Autodesk Inventor part; units mm, degrees
ref_plane "Work Plane3" through (0, 22.5, 0) normal (0, 1, 0) x (1, 0, 0)
ref_plane "YZ Plane" through (0, 0, 0) normal (1, 0, 0) x (0, 1, 0)
ref_plane "XZ Plane" through (0, 0, 0) normal (0, 1, 0) x (-1, 0, 0)
sketch "Sketch1" plane through (0, 0, 0) normal (0, 1, 0) x (-1, 0, 0)
  line L0 (-67.5, 75) -> (67.5, 75)
  line L1 (67.5, 75) -> (67.5, -75)
  line L2 (67.5, -75) -> (-67.5, -75)
  line L3 (-67.5, -75) -> (-67.5, 75)
  line L4 (-67.5, 75) -> (67.5, -75) construction
  line L5 (67.5, 75) -> (-67.5, -75) construction
  point P0 (0, 0)
  dimension "d0" = 135
  dimension "d1" = 150
extrude "Extrusion1" add sketch "Sketch1" along normal blind 8
sketch "Sketch3" plane through (0, 8, 0) normal (0, 1, 0) x (1, 0, 0)
  line L0 (-67.5, -75) -> (67.5, -75)
  line L1 (67.5, -75) -> (67.5, 75)
  line L2 (67.5, 75) -> (-67.5, 75)
  line L3 (-67.5, 75) -> (-67.5, -75)
  line L4 (62.5, 75) -> (62.5, -70)
  line L5 (-67.5, -75) -> (67.5, -75)
  line L6 (67.5, -75) -> (67.5, 75)
  line L7 (0, 0) -> (0, -83) construction
  line L8 (-62.5, 75) -> (-62.5, -70)
  line L9 (62.5, -70) -> (-62.5, -70)
  dimension "d4" = 5
  dimension "d5" = 5
extrude "Extrusion2" add sketch "Sketch3" along normal blind 20 contours L3 L2 L8 L9 L4 L1 L0
sketch "Sketch4" plane through (67.5, 0, -75) normal (0, 0, -1) x (-1, 0, 0)
  line L0 (135, 0) -> (0, 0)
  line L1 (135, 0) -> (135, 28)
  line L2 (130, 28) -> (135, 28)
  line L3 (130, 8) -> (130, 28)
  line L4 (5, 8) -> (130, 8)
  line L5 (5, 8) -> (5, 28)
  line L6 (0, 28) -> (5, 28)
  line L7 (0, 0) -> (0, 28)
  line L8 (130, 8) -> (5, 8)
  line L9 (5, 8) -> (5, 0)
  line L10 (130, 8) -> (130, 0)
  line L11 (0, 0) -> (135, 0)
  line L12 (0, 0) -> (0, 28)
  line L13 (5, 0) -> (130, 0)
  line L14 (5, 8) -> (130, 8)
  line L15 (5, 4) -> (130, 4)
  line L16 (5, 8) -> (0, 8)
  line L17 (135, 0) -> (0, 0)
  point P0 (67.5, 0)
  dimension "d8" = 0
  dimension "d9" = 4
extrude "Extrusion3" add sketch "Sketch4" along normal blind 20 contours L0 L10 L3 L2 L1 | L0 L9 L15 L10 | L15 L9 L4 L10 | L7 L6 L5 L16
sketch "Sketch6" plane through (67.5, 0, 75) normal (1, 0, 0) x (0, 0, -1)
  line L0 (150, 0) -> (150, 8)
  line L1 (0, 0) -> (0, 28)
  line L2 (170, 18) -> (157, 18)
  line L3 (157, 18) -> (157, 28)
  line L4 (157, 28) -> (170, 28)
  line L5 (170, 28) -> (170, 18)
  line L6 (170, 28) -> (170, 8)
  line L7 (150, 8) -> (170, 8)
  line L8 (0, 28) -> (170, 28)
  point P0 (75, 0)
  dimension "d83" = 10
  dimension "d85" = 10
  dimension "d86" = 0
  dimension "d87" = 13
  dimension "d88" = 0
  dimension "d89" = 0
extrude "Extrusion4" cut sketch "Sketch6" against normal through all
fillet "Fillet1" radius 2 11 edges at (67.5, 0, 0) (67.5, 28, -3.5) (67.5, 14, 75) (0, 28, 75) (0, 0, 75) (-67.5, 28, -3.5) (-67.5, 14, 75) (-67.5, 0, -10) (62.5, 28, -6) (-62.5, 28, -6) (0, 28, 70)
sketch "Sketch11" plane through (-67.5, 9.7, -88) normal (-1, 0, 0) x (0, 0, 1)
  line L0 (9, 17.5) -> (0, 19.5)
  line L1 (0, 19.5) -> (0, 11.5)
  line L2 (0, 11.5) -> (9, 14)
  line L3 (9, 17.5) -> (9, 14)
  line L4 (9, 6) -> (0, 8.5)
  line L5 (0, 0) -> (9, 2.5)
  line L6 (0, 6) -> (0, 0)
  line L7 (9, 6) -> (9, 2.5)
  point P0 (88, -9.7)
sketch "Sketch12" plane through (-67.5, 2, 73) normal (-1, 0, 0) x (0, 0, 1)
  line L0 (-168, 28) -> (-168, 20)
  line L1 (-159, 26) -> (-168, 28)
  line L2 (-159, 26) -> (-159, 22.5)
  line L3 (-168, 20) -> (-159, 22.5)
  line L4 (-168, 17) -> (-168, 8.5)
  line L5 (-159, 14.5) -> (-168, 17)
  line L6 (-159, 14.5) -> (-159, 11)
  line L7 (-168, 8.5) -> (-159, 11)
  line L8 (-168, 0) -> (-168, 16)
  line L9 (-161, 19.2) -> (-161, 27.2)
  line L10 (-161, 27.2) -> (-168, 27.2)
  line L11 (-168, 16) -> (-168, 6)
  line L12 (-159, 17) -> (-168, 17)
  point P0 (-73, -2)
  point P1 (-168, 24)
sketch "Sketch15" plane through (62.5, 6, -75) normal (1, 0, 0) x (0, 0, -1)
  line L0 (0, -6) -> (0, 2)
  line L1 (20, 2) -> (20, -6)
  line L2 (0, 2) -> (20, 2)
  line L3 (0, -6) -> (20, -6)
  point P0 (-75, -6)
extrude "Extrusion8" add sketch "Sketch15" along normal blind 2.5
sketch "Sketch16" plane through (0, 8, 0) normal (0, 1, 0) x (1, 0, 0)
  line L0 (-62.5, -35) -> (-52.5, -35)
  line L1 (-52.5, -35) -> (-52.5, 5)
  line L2 (-52.5, 5) -> (-62.5, 5)
  line L3 (-62.5, 5) -> (-62.5, -35)
  line L4 (62.5, -70) -> (-62.5, -70)
  line L5 (-62.5, -70) -> (-62.5, 82)
  line L6 (51.5, -70) -> (62.5, -70)
  line L7 (62.5, -70) -> (62.5, -30)
  line L8 (62.5, -30) -> (51.5, -30)
  line L9 (51.5, -30) -> (51.5, -70)
  line L10 (62.5, 82) -> (62.5, -70)
  point P0 (0, 0)
  point P1 (-62.5, 95)
  point P2 (62.5, 95)
  dimension "d39" = 35
  dimension "d40" = 0
  dimension "d41" = 10
  dimension "d42" = 40
  dimension "d43" = 0
  dimension "d44" = 0
  dimension "d45" = 40
  dimension "d46" = 11
extrude "Extrusion9" add sketch "Sketch16" along normal blind 16
fillet "Fillet4" radius 1 8 edges at (51.5, 24, 50) (57, 24, 30) (51.5, 16, 30) (-52.5, 24, 15) (-52.5, 16, -5) (-57.5, 24, 35) (-57.5, 24, -5) (-52.5, 16, 35)
sketch "Sketch17" plane through (0, 24, 0) normal (0, 1, 0) x (1, 0, 0)
  circle A0 centre (-59, -25) radius 2.25
  line L0 (-62.5, -34) -> (-62.5, 4)
  line L1 (-53.5, -34) -> (-62.5, -34)
  circle A1 centre (58.5, -57.5) radius 2.25
  line L2 (52.5, -70) -> (52.5, -31)
  line L3 (52.5, -31) -> (62.5, -31)
  line L4 (62.5, -70) -> (50.5, -70)
  point P0 (0, 0)
  dimension "d50" = 4.5
  dimension "d51" = 3.5
  dimension "d52" = 9
  dimension "d53" = 4.5
  dimension "d54" = 6
  dimension "d90" = 12.5
extrude "Extrusion10" cut sketch "Sketch17" against normal blind 12
sketch "Sketch18" plane through (-62.5, 9.7, -88) normal (1, 0, 0) x (0, 0, -1)
  circle A0 centre (-68, 13.3) radius 2.25
  circle A1 centre (-37.2, 13.3) radius 2.25
  line L0 (0, 8.1) -> (0, 14.1)
  line L1 (-37.2, 13.3) -> (-68, 13.3)
  line L2 (-6, 18.3) -> (-160, 18.3)
  line L3 (-158, -1.7) -> (-158, 16.3)
  point P0 (-88, -9.7)
  point P1 (7, 18.3)
  dimension "d60" = 4.5
  dimension "d61" = 4.5
  dimension "d62" = 30.8
  dimension "d64" = 5
  dimension "d67" = 90
extrude "Extrusion11" cut sketch "Sketch18" against normal through all
ref_plane "Work Plane3" through (0, 22.5, 0) normal (0, 1, 0) x (1, 0, 0)
sketch "Sketch21" plane through (0, 22.5, 0) normal (0, 1, 0) x (1, 0, 0)
  circle A0 centre (58.5, -57.5) radius 2.25
  line L0 (54.75, -55.3349) -> (58.5, -53.1699)
  line L1 (58.5, -53.1699) -> (62.25, -55.3349)
  line L2 (62.25, -55.3349) -> (62.25, -59.6651)
  line L3 (62.25, -59.6651) -> (58.5, -61.8301)
  line L4 (58.5, -61.8301) -> (54.75, -59.6651)
  line L5 (54.75, -59.6651) -> (54.75, -55.3349)
  line L6 (-62.5, -35) -> (-62.5, -70)
  line L7 (51.5, -70) -> (51.5, -31)
  circle A1 centre (-59, -25) radius 2.25
  line L8 (-55.25, -27.1651) -> (-59, -29.3301)
  line L9 (-59, -29.3301) -> (-62.75, -27.1651)
  line L10 (-62.75, -27.1651) -> (-62.75, -22.8349)
  line L11 (-62.75, -22.8349) -> (-59, -20.6699)
  line L12 (-59, -20.6699) -> (-55.25, -22.8349)
  line L13 (-55.25, -22.8349) -> (-55.25, -27.1651)
  point P0 (0, 0)
  dimension "d78" = 7.5
  dimension "d79" = 7.5
extrude "Extrusion13" cut sketch "Sketch21" against normal blind 3.15
sketch "Sketch22" plane through (0, 8, 0) normal (0, 1, 0) x (1, 0, 0)
  line L0 (65, 75) -> (65, 95)
  line L1 (-62.5, 95) -> (62.5, 95)
  line L2 (65, 75) -> (67.5, 75)
  line L3 (-62.5, 95) -> (65, 95)
  line L4 (65, 95) -> (65, 75)
  line L5 (65, 75) -> (-62.5, 75)
  line L6 (-62.5, 75) -> (-62.5, 95)
  point P0 (0, 0)
extrude "Extrusion14" cut sketch "Sketch22" against normal blind 4
sketch "Sketch23" plane through (65, 6, -75) normal (1, 0, 0) x (0, 0, -1)
  line L0 (20, -2) -> (0, -2)
  line L1 (0, -6) -> (0, -2)
  line L2 (0, -6) -> (20, -6)
  line L3 (20, -6) -> (20, -2)
  point P0 (-75, -6)
extrude "Extrusion15" cut sketch "Sketch23" against normal up to surface (2.5 mm away)
properties part number "Case_metà1"
CAD build for the part. Positions are in the model's coordinates, mm. A direction names the side the tool comes from. Round coordinates to 2 decimals unless told otherwise and drop trailing zeros. Loops run counter-clockwise (first coordinate to the right, second up) from the corner with the lowest first, then second, coordinate; pieces in that order, holes last. Notation, with made-up numbers: (61.5, -24.75) - (107.5, -24.75) arc R21 ccw to (107.5, 2.25) - close; hole circle Ø10 at (65.5, -26). An arc over 180 degrees is marked (long way). Return JSON: item names as keys, results as strings. Group by question number.
Q1. Band-saw the part on C-C on x = -36.5. Give the cut face in (y, z), plus the area to 3 significant figures.
Q2. Flat gauge pins, fed straight in: pin 1 Ø2.5 at (x, z) = (-59, 25) entering from +Y; pin 2 Ø6 at (x, z) = (52, -10) entering from +Y; pin 3 Ø4 at (x, z) = (60, 57) entering from +Y. Where does each tip first touch, or does it go through?
Q3. Drill centre lines: line 1 along X through (y, z) = (22.9, 25); line 2 along X through (y, z) = (22.9, 57.5); line 3 along Z through (x, y) = (-57, 19.25). Where is each one in solid material? Low to high. Write a range as [from, to].
Q4. Tool access for faces 4 (the face through (-52.5, 15, 15)), 5 (the face through (-59, 12, 25)), 6 (the face through (56.8, 19.35, 59.4)): list every direction of +Z, -Z, +X, -X, +Y, -Y with a clear straight run to the whole face (end or side of a thin tool).
Q5. Two-plate mould, pull along Y, no slides. Class faces 1 (the face through (-67.5, 14, -10)), 2 (the face through (-1, 4, -85)), 3 (the face through (56.8, 22.5, 59.4)): +Y half, -Y half, draft (parallel to the pull), parting line (faces both ways), or undercut.
Q6. Band-saw the part on B-B on y = 10. Give the cut face in (x, z), plus the area to 3 significant figures.
Q7. Band-saw the part on A-A on z = -20. Give the cut face in (x, y), plus the area to 3 significant figures.
Solutions:
{
 "1": {"outline": "(0, -95) - (4, -95) - (4, -75) - (8, -75) - (8, 70) - (26, 70) arc R2 ccw to (28, 72) - (28, 73) arc R2 ccw to (26, 75) - (2, 75) arc R2 ccw to (0, 73) - close", "area": "1,380 mm^2"},
 "2": {"pin 1": "stops at y = 12", "pin 2": "stops at y = 8", "pin 3": "stops at y = 24"},
 "3": {"line 1": "x = [-67.5, -61.25], [-56.75, -52.5], [62.5, 67.5]", "line 2": "x = [-67.5, -62.5], [51.5, 56.25], [60.75, 67.5]", "line 3": "z = [-5, 23.97], [26.03, 35], [70, 75]"},
 "4": {"face 4": "-Z, +Y", "face 5": "+Y", "face 6": "none"},
 "5": {"face 1": "draft", "face 2": "+Y half", "face 3": "undercut"},
 "6": {"outline": "(-67.5, -95) - (-62.5, -95) - (-62.5, -5) - (-53.5, -5) arc R1 ccw to (-52.5, -4) - (-52.5, 34) arc R1 ccw to (-53.5, 35) - (-62.5, 35) - (-62.5, 70) - (51.5, 70) - (51.5, 31) arc R1 ccw to (52.5, 30) - (62.5, 30) - (62.5, -95) - (67.5, -95) - (67.5, 73) arc R2 ccw to (65.5, 75) - (-65.5, 75) arc R2 ccw to (-67.5, 73) - close", "area": "3,160 mm^2"},
 "7": {"outline": "(-67.5, 2) arc R2 ccw to (-65.5, 0) - (65.5, 0) arc R2 ccw to (67.5, 2) - (67.5, 26) arc R2 ccw to (65.5, 28) - (64.5, 28) arc R2 ccw to (62.5, 26) - (62.5, 8) - (-62.5, 8) - (-62.5, 20.75) - (-67.5, 20.75) - close; (-67.5, 25.25) - (-62.5, 25.25) - (-62.5, 26) arc R2 ccw to (-64.5, 28) - (-65.5, 28) arc R2 ccw to (-67.5, 26) - close", "area": "1,250 mm^2"}
}
